The listing builds one solid part. Answer for the finished solid, in the listing's coordinates (mm). A direction names the side the tool comes from. Round coordinates to 2 decimals unless told otherwise and drop trailing zeros. Loops run counter-clockwise (first coordinate to the right, second up) from the corner with the lowest first, then second, coordinate; pieces in that order, holes last. Notation, with made-up numbers: (-35.5, 24.25) -> (-13.5, 24.25) arc R5 ccw to (-13.5, 29.25) -> close; hole circle Ø5 at (51.25, 31). An arc over 180 degrees is marked (long way). Write each question's results on one line, items separated by ' | '. Start each with the question number.
(1) Determine the mould class of faces 3 (the face through (-0.49, -12.69, -1.27)), 4 (the face through (0, 32, -1.5)), 5 (the face through (13.813, 27.145, -0.021)), 6 (the face through (24.5, -18.19, -0.02)) for opening direction X: released by +X, released by -X, zero draft, split by the parting line, or undercut.
(2) The part is cut by section D-D (y = 63.5). Determine the outline of the cut face in (x, z), plus the area to 3 significant figures.
(3) The part is cut by section B-B (x = -2). Determine the outline of the cut face in (y, z).
(4) The part is cut by section C-C (y = -1). Determine the outline of the cut face in (x, z).
(5) Straight lines are drawn through the part: probe 1 along Y at (x, z) = (-12.7, 0.7); probe 2 along X at (y, z) = (36.5, 0.55). For each, find the intervals that lie inside material, in ascending order.
(6) Flat-ended cylindrical pins translate along their axes: pin 1 (4 mm diameter, centred on x = 0, y = 57.15, fed in from +Z); pin 2 (5 mm diameter, centred on x = 12.7, y = 38.1, fed in from +Z). Find the tip coordinate at first contact, or state that the pin passes through.
(7) The part is cut by section A-A (y = 38.1). Determine the outline of the cut face in (x, z).
(8) For faces 1 (the face through (0, -6.363, 0)), 2 (the face through (12, -19.05, 0)), determine the directions among +Z, -Z, +X, -X, +Y, -Y from which every point of the face is accessible in a straight line to the end or side of a thin tool.
```python
from build123d import *

# Parameters (mm, degrees)
SKETCH1_R           = 12.7
SKETCH1_R_2         = 3.175
SKETCH1_R_3         = 2.07
BOSS_EXTRUDE1_DEPTH = 1.5
FILLET1_R           = 3.000000096
CUT_EXTRUDE1_START  = -3
CUT_EXTRUDE1_DEPTH  = 3
BOSS_EXTRUDE3_START = -2.54
BOSS_EXTRUDE3_DEPTH = 2.54


with BuildPart() as part:
    # Sketch1 → Boss-Extrude1 (new, symmetric)
    with BuildSketch(Plane.XY):
        Polygon((-19.05, 82.55), (19.05, 82.55), (25.4, 57.15), (25.4, -19.05), (-25.4, -19.05), (-25.4, 57.15), align=None)
        Circle(SKETCH1_R, mode=Mode.SUBTRACT)
        with Locations((-19.05, -12.7)):
            Circle(SKETCH1_R_2, mode=Mode.SUBTRACT)
        with Locations((19.05, 12.7)):
            Circle(SKETCH1_R_2, mode=Mode.SUBTRACT)
        with Locations((-19.05, 12.7)):
            Circle(SKETCH1_R_3, mode=Mode.SUBTRACT)
        with Locations((19.05, -12.7)):
            Circle(SKETCH1_R_3, mode=Mode.SUBTRACT)
        with Locations((0, 57.15)):
            Circle(SKETCH1_R_2, mode=Mode.SUBTRACT)
        with Locations((12.7, 25.4)):
            Circle(SKETCH1_R_3, mode=Mode.SUBTRACT)
        with Locations((12.7, 38.1)):
            Circle(SKETCH1_R_3, mode=Mode.SUBTRACT)
        with Locations((12.7, 50.8)):
            Circle(SKETCH1_R_3, mode=Mode.SUBTRACT)
        with Locations((12.7, 63.5)):
            Circle(SKETCH1_R_3, mode=Mode.SUBTRACT)
        with Locations((12.7, 76.2)):
            Circle(SKETCH1_R_3, mode=Mode.SUBTRACT)
        with Locations(Location((-12.7, 25.4, 0), (0, 0, 180))):
            Circle(SKETCH1_R_3, mode=Mode.SUBTRACT)
        with Locations(Location((-12.7, 38.1, 0), (0, 0, 180))):
            Circle(SKETCH1_R_3, mode=Mode.SUBTRACT)
        with Locations(Location((-12.7, 50.8, 0), (0, 0, 180))):
            Circle(SKETCH1_R_3, mode=Mode.SUBTRACT)
        with Locations(Location((-12.7, 63.5, 0), (0, 0, 180))):
            Circle(SKETCH1_R_3, mode=Mode.SUBTRACT)
        with Locations(Location((-12.7, 76.2, 0), (0, 0, 180))):
            Circle(SKETCH1_R_3, mode=Mode.SUBTRACT)
    extrude(amount=BOSS_EXTRUDE1_DEPTH, both=True)

    # Fillet1
    fillet1_edges = [part.edges().sort_by_distance(p)[0] for p in [
        (-19.05, 82.55, 0),
        (19.05, 82.55, 0),
        (25.4, 57.15, 0),
        (25.4, -19.05, 0),
        (-25.4, -19.05, 0),
        (-25.4, 57.15, 0),
    ]]
    fillet(fillet1_edges, radius=FILLET1_R)

    # Sketch2 → Cut-Extrude1 (cut)
    with BuildSketch(Plane.XY.offset(1.5).offset(CUT_EXTRUDE1_START)):
        with BuildLine():
            Line((5.08, 17.78), (-5.08, 17.78))
            Line((-5.08, 17.78), (-5.08, 11.639742265))
            ThreePointArc((-5.08, 11.639742265), (0, 12.7), (5.08, 11.639742265))
            Line((5.08, 11.639742265), (5.08, 17.78))
        make_face()
        Polygon((0, -17.05), (-1, -19.05), (1, -19.05), align=None)
        Polygon((1, 82.55), (-1, 82.55), (0, 80.55), align=None)
    extrude(amount=CUT_EXTRUDE1_DEPTH, mode=Mode.SUBTRACT)

    # Sketch3 → Boss-Extrude3 (add)
    with BuildSketch(Plane.XY.offset(1.5).offset(BOSS_EXTRUDE3_START)):
        with BuildLine():
            Line((5.08, 17.78), (5.08, 11.639742265))
            ThreePointArc((5.08, 11.639742265), (0, -12.7), (-5.08, 11.639742265))
            Line((-5.08, 11.639742265), (-5.08, 17.78))
            Line((-5.08, 17.78), (5.08, 17.78))
        make_face()
        Polygon((7.347013116, 0), (3.673506558, 6.3627), (-3.673506558, 6.3627), (-7.347013116, 0), (-3.673506558, -6.3627), (3.673506558, -6.3627), align=None, mode=Mode.SUBTRACT)
    extrude(amount=BOSS_EXTRUDE3_DEPTH)


solid = part.part
```
Checked values:
1) face 3: undercut | face 4: zero draft | face 5: undercut | face 6: released by +X
2) outline: (-23.81, -1.5) -> (-14.77, -1.5) -> (-14.77, 1.5) -> (-23.81, 1.5) -> close; (-10.63, -1.5) -> (10.63, -1.5) -> (10.63, 1.5) -> (-10.63, 1.5) -> close; (14.77, -1.5) -> (23.81, -1.5) -> (23.81, 1.5) -> (14.77, 1.5) -> close | area: 118 mm2
3) outline: (-19.05, -1.5) -> (-12.54, -1.5) -> (-12.54, -1.04) -> (-6.36, -1.04) -> (-6.36, 1.5) -> (-19.05, 1.5) -> close; (6.36, -1.04) -> (17.78, -1.04) -> (17.78, -1.5) -> (54.68, -1.5) -> (54.68, 1.5) -> (6.36, 1.5) -> close; (59.62, -1.5) -> (82.55, -1.5) -> (82.55, 1.5) -> (59.62, 1.5) -> close
4) outline: (-25.4, -1.5) -> (-12.66, -1.5) -> (-12.66, -1.04) -> (-6.77, -1.04) -> (-6.77, 1.5) -> (-25.4, 1.5) -> close; (6.77, -1.04) -> (12.66, -1.04) -> (12.66, -1.5) -> (25.4, -1.5) -> (25.4, 1.5) -> (6.77, 1.5) -> close
5) probe 1: y = -19.05 to 23.33, 27.47 to 36.03, 40.17 to 48.73, 52.87 to 61.43, 65.57 to 74.13, 78.27 to 82.55 | probe 2: x = -25.4 to -14.01, -11.39 to 11.39, 14.01 to 25.4
6) pin 1: passes through | pin 2: stops at z = 1.5
7) outline: (-25.4, -1.5) -> (-14.77, -1.5) -> (-14.77, 1.5) -> (-25.4, 1.5) -> close; (-10.63, -1.5) -> (10.63, -1.5) -> (10.63, 1.5) -> (-10.63, 1.5) -> close; (14.77, -1.5) -> (25.4, -1.5) -> (25.4, 1.5) -> (14.77, 1.5) -> close
8) face 1: +Z, -Z | face 2: +Z, -Z, +X, -X, -Y
